Build history of the part. All positions in model axes, mm. Face numbers are marked on the shaded views. A direction names the side the tool comes from. Coordinates: 2 decimals unless noted, no trailing zeros. Loops run counter-clockwise (first coordinate to the right, second up) from the corner with the lowest first, then second, coordinate; pieces in that order, holes last.
Item 1: Drill centre lines: line 1 along Y through (x, z) = (0, 0.85); line 2 along Y through (x, z) = (2.75, 1.7); line 3 along X through (y, z) = (-2.25, 1.55). Where is each one in solid material? Low to high.
Item 2: Mould opens along Y. For the marked faces 1, 2 and 3 say: released by +Y, released by -Y, zero draft, split by the parting line, or undercut.
Item 3: Cut at C-C (y = -4.25). List the corners of the cut face in (x, z).
Item 4: Cut at D-D (x = -3.5). List the corners of the cut face in (y, z).
Item 5: Flat gauge pins, fed straight in: pin 1 (1.5 mm diameter, centred on y = -3.5, z = 2.5, fed in from -X); pin 2 (1.2 mm diameter, centred on y = -0.5, z = 2.5, fed in from +X); pin 3 (1 mm diameter, centred on x = -3.5, y = -5, fed in from +Z); pin 4 (2.5 mm diameter, centred on x = 0, y = 0, fed in from -Z). Where does each tip first touch, or does it go through?
Item 6: Cut at B-B (z = 2.35). List the corners of the cut face in (x, y), and give its area (3 significant figures).
Item 7: Cut at A-A (y = 0). List the corners of the cut face in (x, z), and give its area (3 significant figures).
Item 8: 3-axis set-ups, long thin cutter, end or side, ignore diameter. For the marked faces 4 and 5: which of +Z, -Z, +X, -X, +Y, -Y reach the whole face in a straight line?
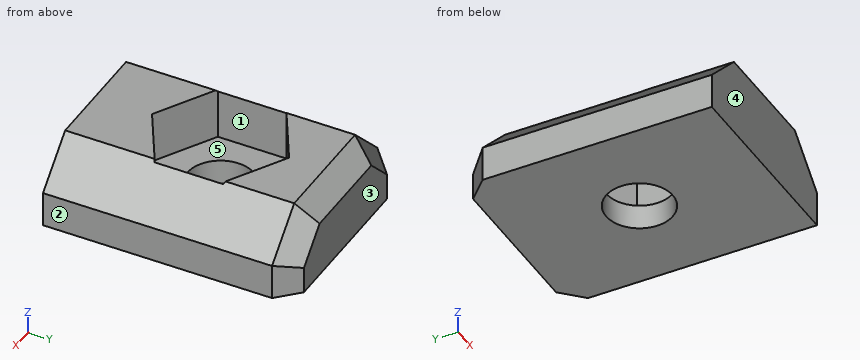
from build123d import *

# Parameters (mm, degrees)
F1_DEPTH = 6
F2_R     = 1.6
F3_DEPTH = 3.7
F5_SIZE2 = 2
F5_SIZE  = 2
F6_DEPTH = 2.5
F7_SIZE  = 1


with BuildPart() as f1:
    # F0 (on Front) → F1 (new body, symmetric)
    with BuildSketch(Plane.XZ):
        Polygon((-4.75, 0), (0, 0), (4.75, 0), (4.75, 3.7), (-4.75, 3.7), align=None)
    extrude(amount=F1_DEPTH, both=True)

    # F2 (on face) → F3 (cut, through all)
    with BuildSketch(Plane.XY.offset(3.7)):
        Circle(F2_R)
    extrude(amount=-F3_DEPTH, mode=Mode.SUBTRACT)

    # F5
    f5_edges = [f1.edges().sort_by_distance(p)[0] for p in [
        (-4.75, 0, 3.7),
        (4.75, 0, 3.7),
    ]]
    chamfer(f5_edges, length=F5_SIZE, length2=F5_SIZE2)

    # F4 (on face) → F6 (cut)
    with BuildSketch(Plane.XY.offset(3.7)):
        Polygon((2.85, -1.6454482672), (2.85, 1.6454482672), (0, 3.2908965344), (-2.85, 1.6454482672), (-2.85, -1.6454482672), (0, -3.2908965344), align=None)
    extrude(amount=-F6_DEPTH, mode=Mode.SUBTRACT)

    # F7
    f7_edges = [f1.edges().sort_by_distance(p)[0] for p in [
        (3.75, 6, 2.7),
        (-3.75, 6, 2.7),
        (-4.75, 6, 0.85),
        (4.75, 6, 0.85),
        (0, 6, 3.7),
    ]]
    chamfer(f7_edges, length=F7_SIZE)


solid = f1.part
Filled sheet:
1. line 1: y = -6 to -1.6, 1.6 to 6
1. line 2: y = -6 to -1.7, 1.7 to 6
1. line 3: x = -4.75 to -1.8, 1.8 to 4.75
2. face 1: undercut
2. face 2: zero draft
2. face 3: released by +Y
3. outline: (-4.75, 0) - (4.75, 0) - (4.75, 1.7) - (2.75, 3.7) - (-2.75, 3.7) - (-4.75, 1.7) - close
4. outline: (-6, 0) - (6, 0) - (6, 1.54) - (5, 2.95) - (-6, 2.95) - close
5. pin 1: stops at x = -4.7
5. pin 2: stops at x = 4.55
5. pin 3: stops at z = 3.45
5. pin 4: passes through
6. outline: (-4.1, -6) - (4.1, -6) - (4.1, 5) - (2.69, 6) - (-2.69, 6) - (-4.1, 5) - close; hole (-2.85, -1.65) - (0, -3.29) - (2.85, -1.65) - (2.85, 1.65) - (0, 3.29) - (-2.85, 1.65) - close
6. area: 68.8 mm2
7. outline: (-4.75, 0) - (-1.6, 0) - (-1.6, 1.2) - (-2.85, 1.2) - (-2.85, 3.6) - (-4.75, 1.7) - close; (1.6, 0) - (4.75, 0) - (4.75, 1.7) - (2.85, 3.6) - (2.85, 1.2) - (1.6, 1.2) - close
7. area: 13.1 mm2
8. face 4: +Z, -Z, +X, -X, -Y
8. face 5: +Z
